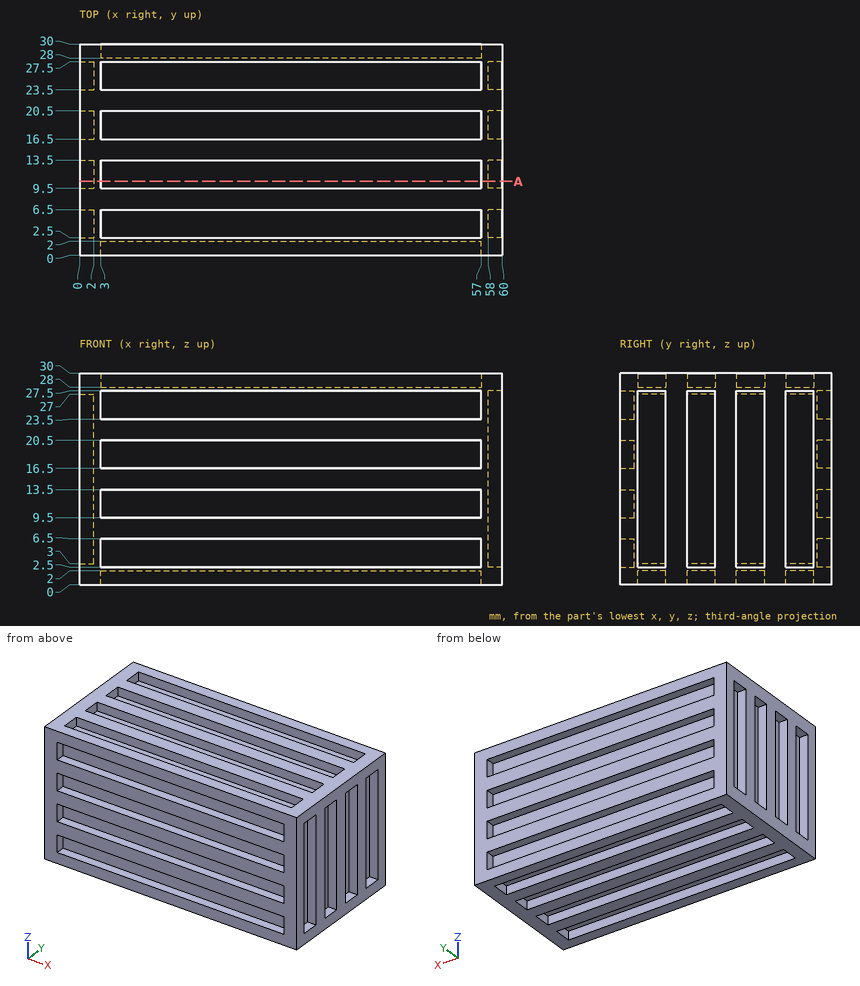
The figure shows three views and two pictorial views of one solid part (mm, origin at its lowest corner). Answer the questions. Round coordinates to 2 decimals unless told otherwise and drop trailing zeros. Order: outer loops, then holes, each group sorted by start corner. A loop starts at its lowest first (then second) coordinate and runs counter-clockwise, first axis right, second up. Notation, with made-up numbers: M 25.25,31.5 L 79.25,31.5 A18 cw 79.25,49.5 Z; hole C 7.25,85.25 d5. An arc over 180 degrees is marked long. Answer in a Markdown table with one row per item. Add a question column.
1) Flat-ended cylindrical pins translate along their axes: pin 1 Ø12 at (x, y) = (37.5, 14.5) entering from -Z; pin 2 Ø1 at (y, z) = (12, 8) entering from -X. Find the tip coordinate at first contact, or state that the pin passes through.
2) The part is cut by section A-A on y = 10.5. Determine the outline of the cut face in (x, z).
3) Consider line 1 along Y through (x, z) = (58.5, 13.75); line 2 along X through (y, z) = (28.25, 11.5); line 3 along Z through (x, y) = (41, 5). Determine where each line is inside the solid, lowest interval first. Write a range as from..to.
Findings below:
| question | item | result |
|---|---|---|
| 1 | pin 1 | stops at z = 0 |
| 1 | pin 2 | stops at x = 2 |
| 2 | outline | M 0,0 L 3,0 L 3,2 L 57,2 L 57,0 L 60,0 L 60,2.5 L 58,2.5 L 58,27.5 L 60,27.5 L 60,30 L 57,30 L 57,28 L 3,28 L 3,30 L 0,30 L 0,27 L 2,27 L 2,3 L 0,3 Z |
| 3 | line 1 | y = 0..2.5, 6.5..9.5, 13.5..16.5, 20.5..23.5, 27.5..30 |
| 3 | line 2 | x = 0..3, 57..60 |
| 3 | line 3 | z = 2..28 |
